from build123d import *

# Parameters (mm, degrees)
SKETCH_1_R          = 2.5
EXTRUDE_1_DEPTH     = 18
SKETCH_2_R          = 4.2
EXTRUDE_2_DEPTH     = 2.9
FILLET_1_R          = 2
CUT_EXTRUDE_1_DEPTH = 2


with BuildPart() as part:
    # 草图1 → 凸台-拉伸1 (new body)
    with BuildSketch(Plane.XY):
        Circle(SKETCH_1_R)
    extrude(amount=EXTRUDE_1_DEPTH)

    # 草图2 → 凸台-拉伸2 (add)
    with BuildSketch(Plane(origin=(0, 0, 0), x_dir=(-1, 0, 0), z_dir=(0, 0, -1))):
        Circle(SKETCH_2_R)
    extrude(amount=EXTRUDE_2_DEPTH)

    # 圆角1
    fillet_1_edges = [part.edges().sort_by_distance(p)[0] for p in [
        (4.2, 0, -2.9),
    ]]
    fillet(fillet_1_edges, radius=FILLET_1_R)

    # 草图3 → 切除-拉伸1 (cut)
    with BuildSketch(Plane(origin=(0, 0, -2.9), x_dir=(-1, 0, 0), z_dir=(0, 0, -1))):
        Polygon((-0.707106781, 0.707106781), (-0.707106781, 6.006401657), (0.707106781, 6.006401657), (0.707106781, 0.707106781), (6.006401657, 0.707106781), (6.006401657, -0.707106781), (0.707106781, -0.707106781), (0.707106781, -6.006401657), (-0.707106781, -6.006401657), (-0.707106781, -0.707106781), (-6.006401657, -0.707106781), (-6.006401657, 0.707106781), align=None)
    extrude(amount=-CUT_EXTRUDE_1_DEPTH, mode=Mode.SUBTRACT)


solid = part.part
Verification items for the finished model (mm, model axes). A direction names the side the tool comes from. Coordinates: 2 decimals unless noted, no trailing zeros. Write each loop counter-clockwise with the first axis right and the second up, starting at its lowest first coordinate (ties: lowest second). Pieces come first, ordered by that corner, then holes. Notation, with made-up numbers: M 51.25,-1.75 L 79.25,-1.75 A26 ccw 79.25,25.25 Z; hole C -30.5,75.25 d7. An arc over 180 degrees is marked long. Use CSV: the item, a comma, the result in double quotes.
Q1. Set-up check for faces 4 (the flat face through (-0.707, 2, -2)), 5 (the cylindrical face through (-0.54, -2.44, 8.87)), 6 (the flat face through (2, -0.707, -2)): record each of +Z, -Z, +X, -X, +Y, -Y from which the full face is reachable in a straight line by a thin tool's end or side.
Computed values:
face 4,"-Z, +Y, -Y"
face 5,"+Z"
face 6,"-Z, +X, -X"
Q2. Mould release check, pull along Y, two halves, no side actions. Record for faces 1 (the flat face through (0, 0, -0.9)), 2 (the cylindrical face through (-4.006, 1.262, -0.444)), 3 (the flat face through (-0.707, -2, -2)): pulls with the +Y half, pulls with the -Y half, needs draft (parallel to the pull), parting line crosses it, or undercut.
Computed values:
face 1,"undercut"
face 2,"parting line crosses it"
face 3,"needs draft"
Q3. Section check B-B, the plane z = 16.75. Enter the section's corners in (x, y).
Computed values:
outline,"C 0,0 d5"
Q4. Thickness scan on line 1 along Z through (x, y) = (3.75, -0.25); line 2 along Y through (x, z) = (0, 11.5); line 3 along Z through (x, y) = (-2, 3.25). Record the ranges inside material, lowest first. Write a range as [from, to].
Computed values:
line 1,"[-0.9, 0]"
line 2,"[-2.5, 2.5]"
line 3,"[-2.08, 0]"
Q5. Go/stop test with flat-tipped pins: P1, Ø2, axis at y = 2, z = -1.5, coming from the -X side; P2, Ø0.6, axis at x = -2, z = -2, coming from the +Y side; P3, Ø0.6, axis at y = -3, z = -2, coming from the +X side. Record where each tip stops, or that it passes through.
Computed values:
P1,"x = -4.05"
P2,"y = 3.57"
P3,"x = 2.86"
Q6. Section check A-A, the plane x = 0. Enter the section's corners in (y, z).
Computed values:
outline,"M -4.2,-0.9 L 4.2,-0.9 L 4.2,0 L 2.5,0 L 2.5,18 L -2.5,18 L -2.5,0 L -4.2,0 Z"
